from build123d import *

# Parameters (mm, degrees)
BOSS_EXTRU_1_DEPTH           = 260
ENL_V_MAT_EXTRU_1_DEPTH      = 261.096136073
ENL_V_MAT_EXTRU_1_DEPTH_BACK = 261.096136073
ESQUISSE2_R                  = 2.5
ESQUISSE3_R                  = 2
BOSS_EXTRU_2_DEPTH           = 20


with BuildPart() as part:
    # Esquisse1 → Boss.-Extru.1 (new body)
    with BuildSketch(Plane.XY):
        with BuildLine():
            Line((-3.249615362, 3.8), (3.249615362, 3.8))
            ThreePointArc((3.249615362, 3.8), (0, -5), (-3.249615362, 3.8))
        make_face()
    extrude(amount=BOSS_EXTRU_1_DEPTH)

    # Esquisse2 → Enlèv. mat.-Extru.1 (cut, two sides: drawn at the far end of the back side and taken through both)
    with BuildSketch(Plane(origin=(0, 0, 0), x_dir=(0, 0, -1), z_dir=(1, 0, 0)).offset(-ENL_V_MAT_EXTRU_1_DEPTH_BACK)):
        with Locations((-255, 0)):
            Circle(ESQUISSE2_R)
    extrude(amount=ENL_V_MAT_EXTRU_1_DEPTH + ENL_V_MAT_EXTRU_1_DEPTH_BACK, mode=Mode.SUBTRACT)

    # Esquisse3 → Boss.-Extru.2 (add, symmetric)
    with BuildSketch(Plane(origin=(0, 0, 0), x_dir=(0, 0, -1), z_dir=(1, 0, 0))):
        with Locations(Location((-224.038713001, 0, 0), (0, 0, 180))):
            Circle(ESQUISSE3_R)
    extrude(amount=BOSS_EXTRU_2_DEPTH, both=True)


solid = part.part
Work out the finished part from the listing and answer in its coordinate system (mm). A direction names the side the tool comes from. Give positions to 0.01 mm unless a question says otherwise; leave off trailing zeros. Order: outer loops, then holes, each group sorted by start corner. A loop starts at its lowest first (then second) coordinate and runs counter-clockwise, first axis right, second up. Notation, with made-up numbers: M 40,-0.5 L 44,-0.5 A19 cw 44,27.5 Z; hole C 26.5,-1.5 d9. An arc over 180 degrees is marked long. Return JSON: item names as keys, results as strings.
Q1. Find the intervals of material crossed by line 1 along Y through (x, z) = (-0.25, 255); line 2 along Z through (x, y) = (2.25, 0); line 3 along X through (y, z) = (0, 147), in increasing order. Write a range as [from, to].
Answer below:
{"line 1": "y = [-4.99, -2.5], [2.5, 3.8]", "line 2": "z = [0, 252.5], [257.5, 260]", "line 3": "x = [-5, 5]"}
Q2. Each of these flat-tipped pins is pushed along its axis until it touches: pin 1 (1 mm diameter, centred on y = -3.5, z = 140.5, fed in from +X); pin 2 (4 mm diameter, centred on x = 8, y = 2.5, fed in from +Z); pin 3 (5 mm diameter, centred on y = -2, z = 217, fed in from -X). Where does it stop, or does it pass through?
Answer below:
{"pin 1": "stops at x = 4", "pin 2": "stops at z = 225.98", "pin 3": "stops at x = -5"}
Q3. The mould has two halves that part along Z. Classify faces 4 (the face through (-20, 0, 224)), 5 (the face through (-0.07, 2.11, 253.66)), 6 (the face through (0, -1, 0)): pulls with the +Z half, pulls with the -Z half, needs draft (parallel to the pull), parting line crosses it, or undercut.
Answer below:
{"face 4": "needs draft", "face 5": "undercut", "face 6": "pulls with the -Z half"}
Q4. Find section A-A, the plane y = 0. Write down the section's boundary in (x, z), and give its area (3 significant figures).
Answer below:
{"outline": "M -20,222.04 L -5,222.04 L -5,0 L 5,0 L 5,222.04 L 20,222.04 L 20,226.04 L 5,226.04 L 5,252.5 L -5,252.5 L -5,226.04 L -20,226.04 Z; M -5,257.5 L 5,257.5 L 5,260 L -5,260 Z", "area": "2,670 mm^2"}
Q5. Find section D-D, the plane x = -16.5. Write down the section's boundary in (y, z).
Answer below:
{"outline": "C 0,224.04 d4"}
Q6. Find section B-B, the plane z = 255. Write down the section's boundary in (x, y).
Answer below:
{"outline": "M -4.33,-2.5 A5 ccw 4.33,-2.5 Z; M -4.33,2.5 L 4.33,2.5 A5 ccw 3.25,3.8 L -3.25,3.8 A5 ccw Z"}
Q7. Which of the six approach directions +Z, -Z, +X, -X, +Y, -Y give full straight-line access (tool end or side, diameter ignored) to faces 1 (the face through (12.399, 0.766, 225.886)), 2 (the face through (-12.183, 0.766, 225.886)), 3 (the face through (0, 3.8, 128))?
Answer below:
{"face 1": "+X", "face 2": "-X", "face 3": "+Z, -Z, +X, -X, +Y"}
Q8. Find section C-C, the plane z = 89.5. Write down the section's boundary in (x, y), and give its area (3 significant figures).
Answer below:
{"outline": "M -3.25,3.8 A5 ccw long 3.25,3.8 Z", "area": "73.2 mm^2"}
